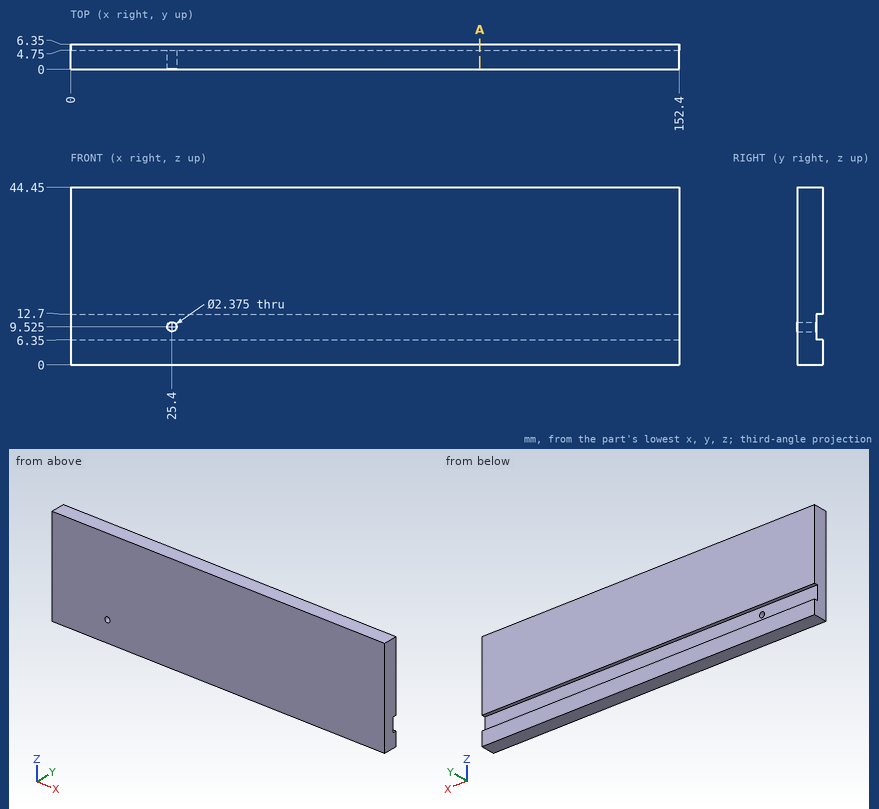
Geometry check sheet. Reference: drawing and pictorial views, mm from the part's lowest x, y, z. Give positions to 0.01 mm unless a question says otherwise; leave off trailing zeros. Order: outer loops, then holes, each group sorted by start corner. A loop starts at its lowest first (then second) coordinate and runs counter-clockwise, first axis right, second up. Notation, with made-up numbers: (70.5, -13) -> (109.5, -13) arc R34 cw to (109.5, 21) -> close; hole circle Ø2 at (-28, 29). An arc over 180 degrees is marked (long way). Write each question's results on one line, items separated by ' | '. Start each with the question number.
(1) Gauge pin test, flat end, axial feed: P1, Ø2.5, axis at x = 25.4, z = 9.525, coming from the +Y side. Record the tip position at first contact, or that the pin passes through.
(2) Sectioned sample at A-A (x = 102.5). Enter the section's corners in (y, z), plus the area to 3 significant figures.
(3) Scan lines: line 1 (Z direction, x = 39, y = 5.5); line 2 (Z direction, x = 25.4, y = 2.45); line 3 (Y direction, x = 24, z = 11). Record each from-to range of solid material in increasing order.
Answer below:
1) P1: y = 4.75
2) outline: (0, 0) -> (6.35, 0) -> (6.35, 6.35) -> (4.75, 6.35) -> (4.75, 12.7) -> (6.35, 12.7) -> (6.35, 44.45) -> (0, 44.45) -> close | area: 272 mm2
3) line 1: 0 to 6.35, 12.7 to 44.45 | line 2: 0 to 8.34, 10.71 to 44.45 | line 3: 0 to 4.75
